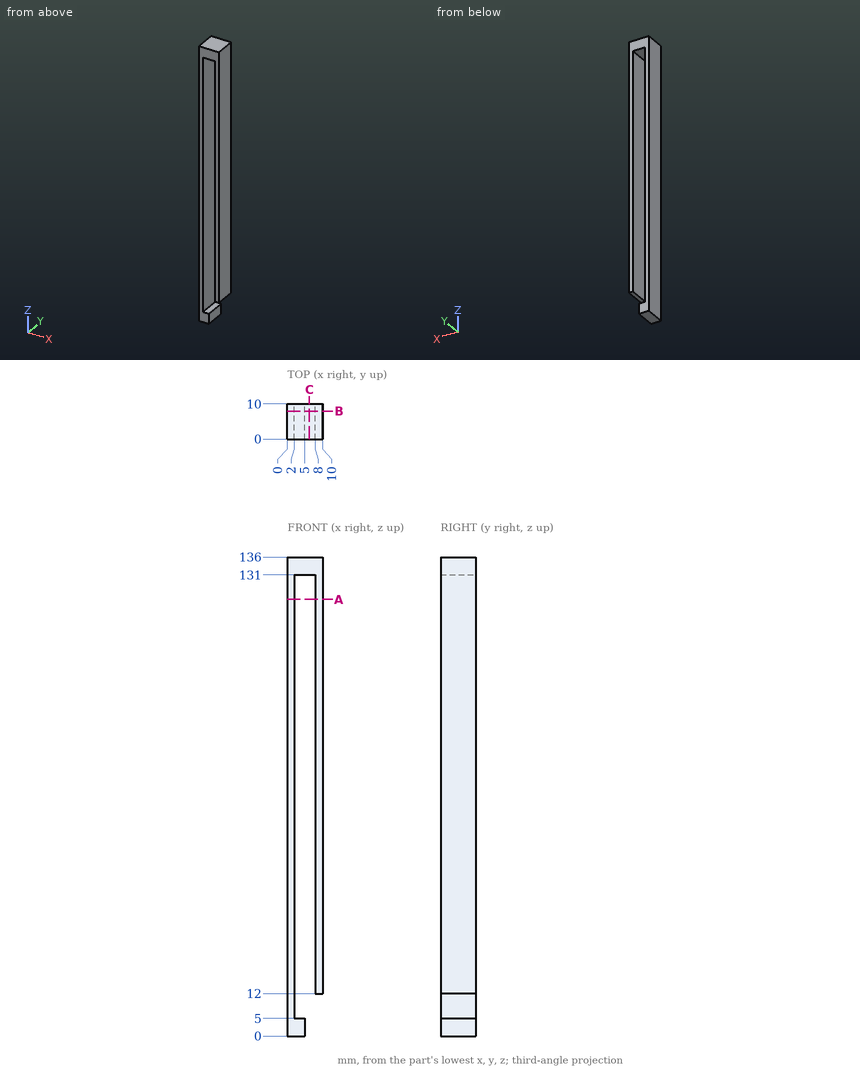
Input: dimensioned drawing with shaded views. Units: mm. Origin: part minimum x, y, z. Coordinates: 2 decimals unless noted, no trailing zeros. Loops run counter-clockwise (first coordinate to the right, second up) from the corner with the lowest first, then second, coordinate; pieces in that order, holes last. Notation, with made-up numbers: M 36,-20.75 L 54,-20.75 A10 cw 54,-3.75 Z; hole C -19,8.25 d2. An arc over 180 degrees is marked long. Use a Markdown table: item, result. Add a question column.
Q1. Section query B-B, the plane y = 8. Return loops of the section in (x, z).
Q2. Material intervals for L1, parallel to X at y = 8, z = 19.5; L2, parallel to Z at x = 3.5, y = 8.75; L3, parallel to Z at x = 6.75, y = 5, sorted ascending.
Q3. Section query C-C, the plane x = 6.25. Return loops of the section in (y, z).
Q4. First-contact query: pin 1 (1.5 mm diameter, centred on x = 6, y = 4, fed in from -Z); pin 2 (6 mm diameter, centred on x = 1.5, y = 1.5, fed in from -Z); pin 3 (0.6 mm diameter, centred on x = 9.5, y = 3, fed in from -Z); pin 4 (2.5 mm diameter, centred on y = 3.5, z = 2.5, fed in from +X). Flat tips, straight axial feed; report the tip coordinate or a pass-through.
Q5. Section query A-A, the plane z = 124. Return loops of the section in (x, y), and give its area (3 significant figures).
Result:
| question | item | result |
|---|---|---|
| 1 | outline | M 0,0 L 5,0 L 5,5 L 2,5 L 2,131 L 8,131 L 8,12 L 10,12 L 10,136 L 0,136 Z |
| 2 | L1 | x = 0 to 2, 8 to 10 |
| 2 | L2 | z = 0 to 5, 131 to 136 |
| 2 | L3 | z = 131 to 136 |
| 3 | outline | M 0,131 L 10,131 L 10,136 L 0,136 Z |
| 4 | pin 1 | stops at z = 131 |
| 4 | pin 2 | stops at z = 0 |
| 4 | pin 3 | stops at z = 12 |
| 4 | pin 4 | stops at x = 5 |
| 5 | outline | M 0,0 L 2,0 L 2,10 L 0,10 Z; M 8,0 L 10,0 L 10,10 L 8,10 Z |
| 5 | area | 40.0 mm2 |
